Can you work these out from the model? Positions are in its coordinate system, mm. Face numbers are marked on the shaded views. A direction names the side the tool comes from. Coordinates: 2 decimals unless noted, no trailing zeros. Order: outer loops, then holes, each group sorted by start corner. A loop starts at its lowest first (then second) coordinate and runs counter-clockwise, first axis right, second up. Notation, with made-up numbers: (26, 48.5) -> (48, 48.5) arc R15 ccw to (48, 70.5) -> close; hole circle Ø8 at (12, 72). An arc over 180 degrees is marked (long way). Answer as CSV lines item,"result".
from build123d import *

# Parameters (mm, degrees)
F0_W     = 127
F0_H     = 38
F1_DEPTH = 58
F2_W     = 58
F2_H     = 6
F3_DEPTH = 11
F4_W     = 58
F4_H     = 6
F5_DEPTH = 11
F6_W     = 36.136753
F6_H     = 7.943855
F7_DEPTH = 200


with BuildPart() as f1:
    # F0 (on Front) → F1 (new body)
    with BuildSketch(Plane.XZ):
        with Locations((63.5, 19)):
            Rectangle(F0_W, F0_H)
    extrude(amount=F1_DEPTH)

    # F2 (on face) → F3 (cut)
    with BuildSketch(Plane.YZ.offset(127)):
        with Locations((-29, 3)):
            Rectangle(F2_W, F2_H)
    extrude(amount=-F3_DEPTH, mode=Mode.SUBTRACT)

    # F4 (on face) → F5 (cut)
    with BuildSketch(Plane(origin=(0, 0, 0), x_dir=(0, -1, 0), z_dir=(-1, 0, 0))):
        with Locations((29, 3)):
            Rectangle(F4_W, F4_H)
    extrude(amount=-F5_DEPTH, mode=Mode.SUBTRACT)

    # F6 (on face) → F7 (cut)
    with BuildSketch(Plane.YZ.offset(127)):
        with Locations((-28.729976, 34.028073)):
            Rectangle(F6_W, F6_H)
    extrude(amount=-F7_DEPTH, mode=Mode.SUBTRACT)


solid = f1.part
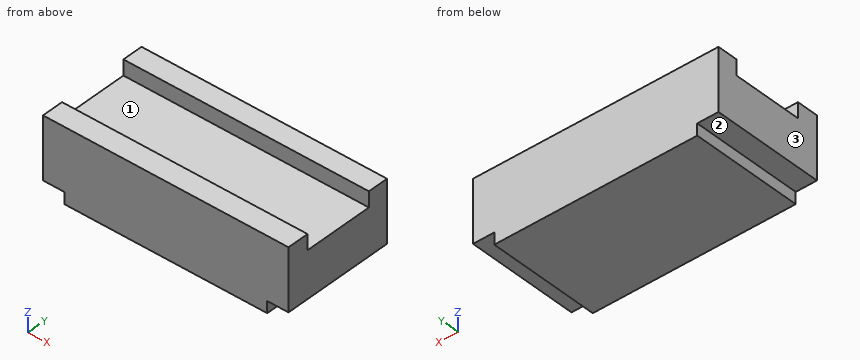
Q1. If I drill on line 1 (Y direction, x = 110.5, z = 34); line 2 (Z direction, x = 71.5, y = -45.5); line 3 (Z direction, x = 7.5, y = -5.5), over which ranges is the centre line in solid material (lowest first)?
Solution:
line 1,"-58 to -46.8, -10.66 to 0"
line 2,"0 to 30.06"
line 3,"6 to 38"
Q2. Which directions (+Z, -Z, +X, -X, +Y, -Y) give clear straight access to the entire face, cutting with the end or side of a thin tool? Please do the marked faces 1, 2 and 3.
Solution:
face 1,"+Z, +X, -X"
face 2,"-Z, -X, +Y, -Y"
face 3,"+Z, -Z, -X, +Y, -Y"
Q3. Imagine slicing it at C-C (z = 3). List the corners of the cut face in (x, y) for me, and give its area (3 significant figures).
Solution:
outline,"(11, -58) -> (116, -58) -> (116, 0) -> (11, 0) -> close"
area,"6,090 mm2"
Q4. For P1, Ø3.5, axis at x = 121.5, y = -20.5, coming from the -Z side; P2, Ø5, axis at y = -17, z = 3, coming from the +X side; P3, Ø1.8, axis at y = -41, z = 2.5, coming from the -X side, each with a flat end and sliding along its axis, tell me the tip position at first contact or that it passes through.
Solution:
P1,"z = 6"
P2,"x = 116"
P3,"x = 11"
Q5. Imagine slicing it at A-A (y = -12). List the corners of the cut face in (x, z) for me.
Solution:
outline,"(0, 6) -> (11, 6) -> (11, 0) -> (116, 0) -> (116, 6) -> (127, 6) -> (127, 30.06) -> (0, 30.06) -> close"
Q6. Imagine slicing it at B-B (x = 48). List the corners of the cut face in (y, z) for me, and give its area (3 significant figures).
Solution:
outline,"(-58, 0) -> (0, 0) -> (0, 38) -> (-10.66, 38) -> (-10.66, 30.06) -> (-46.8, 30.06) -> (-46.8, 38) -> (-58, 38) -> close"
area,"1,920 mm2"
